from build123d import *

# Parameters (mm, degrees)
SKETCH1_R           = 2.125
SKETCH1_R_2         = 1.787095899
SKETCH1_W           = 19.725
SKETCH1_H           = 4
BOSS_EXTRUDE1_DEPTH = 4


with BuildPart() as part:
    # Sketch1 → Boss-Extrude1 (new body)
    with BuildSketch(Plane(origin=(0, 0, 0), x_dir=(1, 0, 0), z_dir=(0, 1, 0))):
        with BuildLine():
            Line((299.8, 24), (299.8, 4))
            Line((299.8, 4), (295.8, 4))
            Line((295.8, 4), (295.8, -16))
            Line((295.8, -16), (299.8, -16))
            Line((299.8, -16), (299.8, -36))
            Line((299.8, -36), (295.8, -36))
            Line((295.8, -36), (295.8, -56))
            Line((295.8, -56), (299.8, -56))
            Line((299.8, -56), (299.8, -76))
            Line((299.8, -76), (275.8, -76))
            Line((275.8, -76), (275.8, -75))
            ThreePointArc((275.8, -75), (259.690872965, -36.109127035), (220.8, -20))
            Line((220.8, -20), (-220.8, -20))
            ThreePointArc((-220.8, -20), (-259.690872965, -36.109127035), (-275.8, -75))
            Line((-275.8, -75), (-275.8, -76))
            Line((-275.8, -76), (-299.8, -76))
            Line((-299.8, -76), (-299.8, -56))
            Line((-299.8, -56), (-295.8, -56))
            Line((-295.8, -56), (-295.8, -36))
            Line((-295.8, -36), (-299.8, -36))
            Line((-299.8, -36), (-299.8, -16))
            Line((-299.8, -16), (-295.8, -16))
            Line((-295.8, -16), (-295.8, 4))
            Line((-295.8, 4), (-299.8, 4))
            Line((-299.8, 4), (-299.8, 24))
            Line((-299.8, 24), (299.8, 24))
        make_face()
        with Locations((285.8, -61)):
            Circle(SKETCH1_R, mode=Mode.SUBTRACT)
        with Locations((285.8, -46)):
            Circle(SKETCH1_R, mode=Mode.SUBTRACT)
        with Locations((-285.8, -46)):
            Circle(SKETCH1_R, mode=Mode.SUBTRACT)
        with Locations((-285.8, -61)):
            Circle(SKETCH1_R, mode=Mode.SUBTRACT)
        with Locations((285.8, -16)):
            Circle(SKETCH1_R, mode=Mode.SUBTRACT)
        with Locations((285.8, -31)):
            Circle(SKETCH1_R, mode=Mode.SUBTRACT)
        with Locations((-285.8, -31)):
            Circle(SKETCH1_R, mode=Mode.SUBTRACT)
        with Locations((-285.8, -16)):
            Circle(SKETCH1_R, mode=Mode.SUBTRACT)
        with Locations((-149.9, -10)):
            Circle(SKETCH1_R, mode=Mode.SUBTRACT)
        with Locations((149.9, -10)):
            Circle(SKETCH1_R, mode=Mode.SUBTRACT)
        with Locations((0, -10)):
            Circle(SKETCH1_R_2, mode=Mode.SUBTRACT)
        with Locations((0, 2)):
            Rectangle(SKETCH1_W, SKETCH1_H, mode=Mode.SUBTRACT)
        with Locations((39.45, 2)):
            Rectangle(SKETCH1_W, SKETCH1_H, mode=Mode.SUBTRACT)
        with Locations((78.87, 2)):
            Rectangle(SKETCH1_W, SKETCH1_H, mode=Mode.SUBTRACT)
        with Locations((118.29, 2)):
            Rectangle(SKETCH1_W, SKETCH1_H, mode=Mode.SUBTRACT)
        with Locations((157.71, 2)):
            Rectangle(SKETCH1_W, SKETCH1_H, mode=Mode.SUBTRACT)
        with Locations((197.13, 2)):
            Rectangle(SKETCH1_W, SKETCH1_H, mode=Mode.SUBTRACT)
        with Locations((236.55, 2)):
            Rectangle(SKETCH1_W, SKETCH1_H, mode=Mode.SUBTRACT)
        with Locations((275.97, 2)):
            Rectangle(SKETCH1_W, SKETCH1_H, mode=Mode.SUBTRACT)
        with Locations((-275.97, 2)):
            Rectangle(SKETCH1_W, SKETCH1_H, mode=Mode.SUBTRACT)
        with Locations((-236.55, 2)):
            Rectangle(SKETCH1_W, SKETCH1_H, mode=Mode.SUBTRACT)
        with Locations((-197.13, 2)):
            Rectangle(SKETCH1_W, SKETCH1_H, mode=Mode.SUBTRACT)
        with Locations((-157.71, 2)):
            Rectangle(SKETCH1_W, SKETCH1_H, mode=Mode.SUBTRACT)
        with Locations((-118.29, 2)):
            Rectangle(SKETCH1_W, SKETCH1_H, mode=Mode.SUBTRACT)
        with Locations((-78.87, 2)):
            Rectangle(SKETCH1_W, SKETCH1_H, mode=Mode.SUBTRACT)
        with Locations((-39.45, 2)):
            Rectangle(SKETCH1_W, SKETCH1_H, mode=Mode.SUBTRACT)
    extrude(amount=BOSS_EXTRUDE1_DEPTH)


solid = part.part
Could you check a few things on this model? Use its own coordinates, in mm. A direction names the side the tool comes from. Coordinates: 2 decimals unless noted, no trailing zeros. Write each loop counter-clockwise with the first axis right and the second up, starting at its lowest first coordinate (ties: lowest second). Pieces come first, ordered by that corner, then holes. Notation, with made-up numbers: (1.5, -37.5) - (54.5, -37.5) arc R27 cw to (54.5, -16.5) - close; hole circle Ø4 at (26.25, 12). An arc over 180 degrees is marked (long way). Write item = value, one per line.
1) Please list where these lines run through material, in increasing order: line 1 (X direction, y = 3.15, z = 10) (3 decimals); line 2 (Z direction, x = 285.8, y = 2.7) (3 decimals); line 3 (Z direction, x = 149.9, y = 3.1) (3 decimals). Write a range as [from, to].
Result set:
line_1 = [-295.8, -152.025], [-147.775, -1.787], [1.787, 147.775], [152.025, 295.8]
line_2 = [-24, -4], [0, 13.875], [18.125, 28.875], [33.125, 43.875], [48.125, 58.875], [63.125, 76]
line_3 = [-24, -4], [0, 7.875], [12.125, 20]
2) Suppose I cut it at C-C on x = -139.5. Please give me the cut outline in (y, z).
Result set:
outline = (0, -24) - (4, -24) - (4, 20) - (0, 20) - close
3) Suppose I cut it at A-A on x = 120.5. Please give me the cut outline in (y, z).
Result set:
outline = (0, -24) - (4, -24) - (4, -4) - (0, -4) - close; (0, 0) - (4, 0) - (4, 20) - (0, 20) - close
4) Will these pins go through, and if not, where does the flat tip stop? pin 1 Ø1.2 at (y, z) = (1.5, 46) entering from -X; pin 2 Ø2.5 at (x, z) = (-285.8, 16) entering from -Y; pin 3 Ø1.2 at (y, z) = (2, -1) entering from +X.
Result set:
pin_1 = -295.8
pin_2 = through
pin_3 = 295.8
5) Suppose I cut it at B-B on y = 1.45. State how many separate pieces and enclosed holes the cut face has, plus the area to 3 significant figures.
Result set:
separate_pieces = 1
enclosed_holes = 26
area = 28,700 mm2
6) For faces 1 (the cylindrical face through (-259.261, 1.972, 35.684)), 2 (the flat face through (4, 4, 3)), which set-ups out of +Z, -Z, +X, -X, +Y, -Y let a thin tool reach every point of the face, with its end or its side?
Result set:
face_1 = +Z, +Y, -Y
face_2 = +Z, -Z, +X, -X, +Y
7) We'd pull the mould along X, two halves only. Please class faces 3 (the flat face through (4, 0, 3)), 4 (the cylindrical face through (260.116, 1.972, 36.539)): +X half, -X half, draft (parallel to the pull), parting line (faces both ways), or undercut.
Result set:
face_3 = draft
face_4 = undercut
